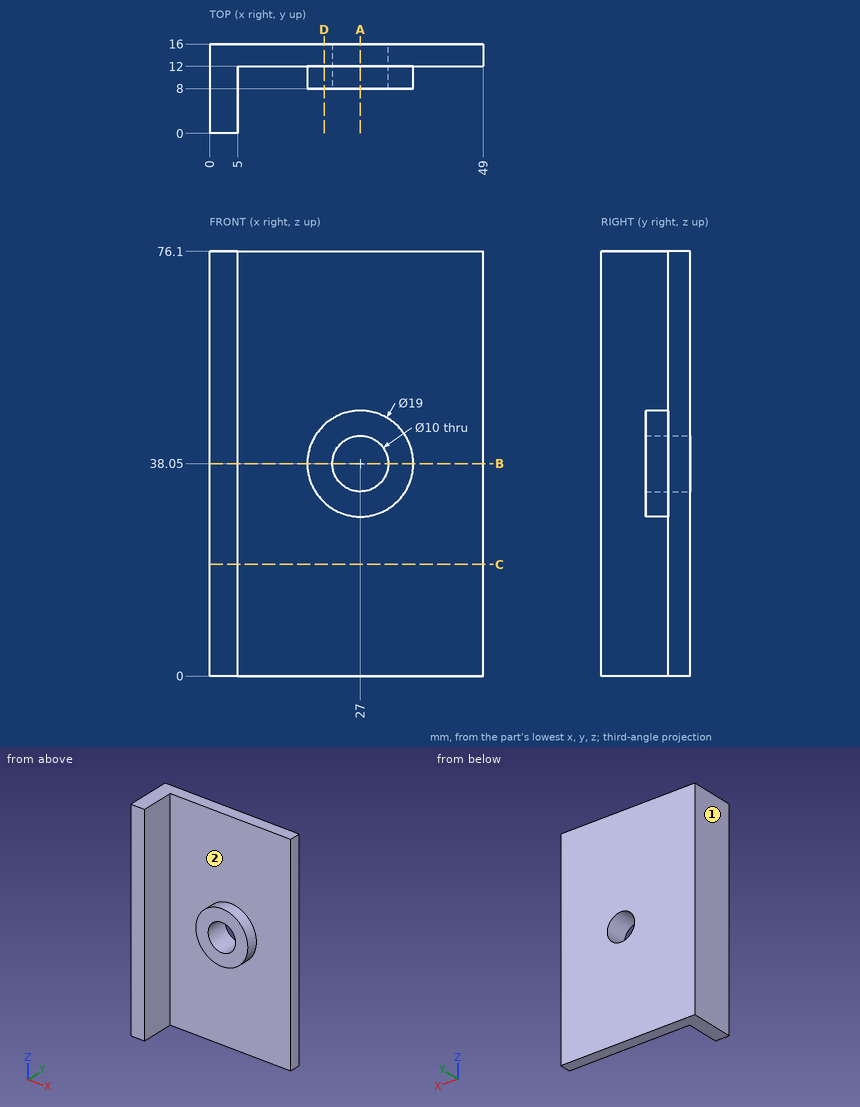
Answer from the drawing. Dimensions are ordinates in mm from the lowest x, y and z of the part. A direction names the side the tool comes from. Give positions to 0.01 mm unless a question says otherwise; leave off trailing zeros. Loops run counter-clockwise (first coordinate to the right, second up) from the corner with the lowest first, then second, coordinate; pieces in that order, holes last.
Item 1: The part is cut by section C-C (z = 20). Write down the section's boundary in (x, y), and give its area (3 significant figures).
Item 2: The part is cut by section A-A (x = 27). Write down the section's boundary in (y, z), and give its area (3 significant figures).
Item 3: For the marked faces 1 and 2, determine the directions among +Z, -Z, +X, -X, +Y, -Y from which every point of the face is accessible in a straight line to the end or side of a thin tool.
Item 4: The part is cut by section D-D (x = 20.5). Write down the section's boundary in (y, z), and give its area (3 significant figures).
Item 5: Find the intervals of material crossed by line 1 along X through (y, z) = (10.75, 40); line 2 along Z through (x, y) = (27, 10.25); line 3 along Z through (x, y) = (27, 13.75), in increasing order.
Item 6: The part is cut by section B-B (z = 38.05). Write down the section's boundary in (x, y).
Item 7: Each of these flat-tipped pins is pushed along its axis until it touches: pin 1 Ø1.5 at (x, z) = (21.5, 35.5) entering from -Y; pin 2 Ø6 at (x, z) = (42.5, 67.5) entering from -Y. Where does it stop, or does it pass through?
Taken from the geometry:
1. outline: (0, 0) - (5, 0) - (5, 12) - (49, 12) - (49, 16) - (0, 16) - close
1. area: 256 mm2
2. outline: (8, 28.55) - (12, 28.55) - (12, 0) - (16, 0) - (16, 33.05) - (8, 33.05) - close; (8, 43.05) - (16, 43.05) - (16, 76.1) - (12, 76.1) - (12, 47.55) - (8, 47.55) - close
2. area: 300 mm2
3. face 1: +Z, -Z, -X, +Y, -Y
3. face 2: -Y
4. outline: (8, 31.12) - (12, 31.12) - (12, 0) - (16, 0) - (16, 76.1) - (12, 76.1) - (12, 44.98) - (8, 44.98) - close
4. area: 360 mm2
5. line 1: x = 0 to 5, 17.7 to 22.4, 31.6 to 36.3
5. line 2: z = 28.55 to 33.05, 43.05 to 47.55
5. line 3: z = 0 to 33.05, 43.05 to 76.1
6. outline: (0, 0) - (5, 0) - (5, 12) - (17.5, 12) - (17.5, 8) - (22, 8) - (22, 16) - (0, 16) - close; (32, 8) - (36.5, 8) - (36.5, 12) - (49, 12) - (49, 16) - (32, 16) - close
7. pin 1: stops at y = 8
7. pin 2: stops at y = 12
